Geometry: final body of the model. Coordinates: model frame, mm. Give positions to 0.01 mm unless a question says otherwise; leave off trailing zeros. Order: outer loops, then holes, each group sorted by start corner. A loop starts at its lowest first (then second) coordinate and runs counter-clockwise, first axis right, second up. Notation, with made-up numbers: (39.25, -18) - (47.25, -18) arc R17 ccw to (47.25, 6) - close; hole circle Ø8 at (45, -36). An arc over 180 degrees is marked (long way). Write item = value, one per line. Start each with the question number.
from build123d import *

# Parameters (mm, degrees)
SKETCH1_R           = 10
SKETCH1_R_2         = 3
BOSS_EXTRUDE1_DEPTH = 5


with BuildPart() as part:
    # Sketch1 → Boss-Extrude1 (new body)
    with BuildSketch(Plane.XY):
        with BuildLine():
            Line((-90, 150), (90, 150))
            ThreePointArc((90, 150), (97.071067812, 147.071067812), (100, 140))
            Line((100, 140), (100, -140))
            ThreePointArc((100, -140), (97.071067812, -147.071067812), (90, -150))
            Line((90, -150), (-90, -150))
            ThreePointArc((-90, -150), (-97.071067812, -147.071067812), (-100, -140))
            Line((-100, -140), (-100, 140))
            ThreePointArc((-100, 140), (-97.071067812, 147.071067812), (-90, 150))
        make_face()
        with Locations((0, 125)):
            Circle(SKETCH1_R, mode=Mode.SUBTRACT)
        with Locations((50, 80)):
            Circle(SKETCH1_R_2, mode=Mode.SUBTRACT)
        with Locations((-50, 80)):
            Circle(SKETCH1_R_2, mode=Mode.SUBTRACT)
        with Locations((-50, -80)):
            Circle(SKETCH1_R_2, mode=Mode.SUBTRACT)
        with Locations((50, -80)):
            Circle(SKETCH1_R_2, mode=Mode.SUBTRACT)
        with BuildLine():
            Line((-0.55, -138.602627944), (-0.55, -139.8))
            Line((-0.55, -139.8), (0.55, -139.8))
            Line((0.55, -139.8), (0.55, -138.602627944))
            ThreePointArc((0.55, -138.602627944), (0, -136.55), (-0.55, -138.602627944))
        make_face(mode=Mode.SUBTRACT)
        with BuildLine():
            Line((-0.55, -107.7), (-0.55, -108.897372056))
            ThreePointArc((-0.55, -108.897372056), (0, -110.95), (0.55, -108.897372056))
            Line((0.55, -108.897372056), (0.55, -107.7))
            Line((0.55, -107.7), (-0.55, -107.7))
        make_face(mode=Mode.SUBTRACT)
        with BuildLine():
            Line((-6.1, -113.35), (-6.1, -134.15))
            ThreePointArc((-6.1, -134.15), (-5.851040764, -134.751040764), (-5.25, -135))
            Line((-5.25, -135), (5.25, -135))
            ThreePointArc((5.25, -135), (5.851040764, -134.751040764), (6.1, -134.15))
            Line((6.1, -134.15), (6.1, -113.35))
            ThreePointArc((6.1, -113.35), (5.851040764, -112.748959236), (5.25, -112.5))
            Line((5.25, -112.5), (-5.25, -112.5))
            ThreePointArc((-5.25, -112.5), (-5.851040764, -112.748959236), (-6.1, -113.35))
        make_face(mode=Mode.SUBTRACT)
    extrude(amount=BOSS_EXTRUDE1_DEPTH)


solid = part.part
Q1. Pull-direction query (X, two-part tool) for faces 1 (the flat face through (1, 2, 0)), 2 (the cylindrical face through (5.38, 133.43, 2.46)), 3 (the cylindrical face through (96.99, 147.15, 2.46)); classes: +X half, -X half, draft (parallel to the pull), parting line (faces both ways), or undercut.
Q2. Section D-D, the plane y = 125. Return the cut outline in (x, z), then the cut area to 3 significant figures.
Q3. Section A-A, the plane y = 80. Return the cut outline in (x, z).
Q4. Material intervals for line 1 along Y through (x, z) = (0, 3.4); line 2 along Y through (x, z) = (-50, 2.05); line 3 along X through (y, z) = (-125.5, 0.8), sorted ascending. Write a range as from..to.
Q5. Section B-B, the plane y = -121. Return the cut outline in (x, z), then the cut area to 3 significant figures.
Q6. Section C-C, the plane x = -50. Return the cut outline in (y, z), then the cut area to 3 significant figures.
The answers:
q1.face_1 = draft
q1.face_2 = undercut
q1.face_3 = +X half
q2.outline = (-100, 0) - (-10, 0) - (-10, 5) - (-100, 5) - close; (10, 0) - (100, 0) - (100, 5) - (10, 5) - close
q2.area = 900 mm²
q3.outline = (-100, 0) - (-53, 0) - (-53, 5) - (-100, 5) - close; (-47, 0) - (47, 0) - (47, 5) - (-47, 5) - close; (53, 0) - (100, 0) - (100, 5) - (53, 5) - close
q4.line_1 = -150..-139.8, -136.55..-135, -112.5..-110.95, -107.7..115, 135..150
q4.line_2 = -150..-83, -77..77, 83..150
q4.line_3 = -100..-6.1, 6.1..100
q5.outline = (-100, 0) - (-6.1, 0) - (-6.1, 5) - (-100, 5) - close; (6.1, 0) - (100, 0) - (100, 5) - (6.1, 5) - close
q5.area = 939 mm²
q6.outline = (-150, 0) - (-83, 0) - (-83, 5) - (-150, 5) - close; (-77, 0) - (77, 0) - (77, 5) - (-77, 5) - close; (83, 0) - (150, 0) - (150, 5) - (83, 5) - close
q6.area = 1,440 mm²
